CAD build for the part. Positions are in the model's coordinates, mm. A direction names the side the tool comes from. Coordinates: 2 decimals unless noted, no trailing zeros. Order: outer loops, then holes, each group sorted by start corner. A loop starts at its lowest first (then second) coordinate and runs counter-clockwise, first axis right, second up. Notation, with made-up numbers: M -31.75,38 L -18.75,38 A21 ccw -18.75,54 Z; hole C 62.5,22 d5. An arc over 180 degrees is marked long. One line per item, written item: value.
from build123d import *

# Parameters (mm, degrees)
F0_W     = 1500
F0_H     = 700
F1_DEPTH = 40
F2_W     = 300
F2_H     = 500
F3_DEPTH = 700
F4_W     = 420
F4_H     = 620
F5_DEPTH = 1328


with BuildPart() as f1:
    # F0 (on Top) → F1 (new body)
    with BuildSketch(Plane.XY):
        with Locations((750, -350)):
            Rectangle(F0_W, F0_H)
    extrude(amount=-F1_DEPTH)

    # F2 (on face) → F3 (join)
    with BuildSketch(Plane(origin=(0, 0, -40), x_dir=(1, 0, 0), z_dir=(0, 0, -1))):
        with Locations((250, 350)):
            Rectangle(F2_W, F2_H)
        with Locations((1250, 350)):
            Rectangle(F2_W, F2_H)
    extrude(amount=F3_DEPTH)

    # F4 (on face) → F5 (cut)
    with BuildSketch(Plane(origin=(100, 0, 0), x_dir=(0, -1, 0), z_dir=(-1, 0, 0))):
        with Locations((350, -390)):
            Rectangle(F4_W, F4_H)
    extrude(amount=-F5_DEPTH, mode=Mode.SUBTRACT)


solid = f1.part
Q1. Pin check, flat tips, straight feed: pin 1 Ø1 at (x, z) = (1127, -99.5) entering from +Y; pin 2 Ø3 at (x, y) = (482, -475) entering from -Z; pin 3 Ø1 at (x, y) = (496, -418.5) entering from +Z. Stop position of each tip, or through.
Recorded:
pin 1: stops at y = -100
pin 2: stops at z = -40
pin 3: stops at z = 0
Q2. Slice it at D-D (x = 338). List the corners of the cut face in (y, z), plus the area to 3 significant figures.
Recorded:
outline: M -700,-40 L -600,-40 L -600,-740 L -100,-740 L -100,-40 L 0,-40 L 0,0 L -700,0 Z; hole M -560,-700 L -140,-700 L -140,-80 L -560,-80 Z
area: 118,000 mm^2
Q3. Which spindle directions (+Z, -Z, +X, -X, +Y, -Y) get a long thin tool onto all of the face, cutting with end or side? Do faces 4 (the face through (740, -700, -20)), 5 (the face through (248, -100, -385)), 6 (the face through (1248, -600, -385)), 7 (the face through (248, -347, -700)), 8 (the face through (1100, -127, -362)). Say none if no direction does.
Recorded:
face 4: +Z, -Z, +X, -X, -Y
face 5: -Z, +X, -X, +Y
face 6: -Z, +X, -X, -Y
face 7: +X, -X
face 8: -Z, +Y, -Y
Q4. Drill centre lines: line 1 along Y through (x, z) = (195.5, -242); line 2 along Z through (x, y) = (267, -293.5); line 3 along Z through (x, y) = (902.5, -162). Where is each one in solid material? Low to high.
Recorded:
line 1: y = -600 to -560, -140 to -100
line 2: z = -740 to -700, -80 to 0
line 3: z = -40 to 0
Q5. Slice it at C-C (y = -542). List the corners of the cut face in (x, z).
Recorded:
outline: M 0,-40 L 100,-40 L 100,-80 L 400,-80 L 400,-40 L 1100,-40 L 1100,-80 L 1400,-80 L 1400,-40 L 1500,-40 L 1500,0 L 0,0 Z; M 100,-740 L 400,-740 L 400,-700 L 100,-700 Z; M 1100,-740 L 1400,-740 L 1400,-700 L 1100,-700 Z
Q6. Slice it at B-B (z = -556). List the corners of the cut face in (x, y).
Recorded:
outline: M 100,-600 L 400,-600 L 400,-560 L 100,-560 Z; M 100,-140 L 400,-140 L 400,-100 L 100,-100 Z; M 1100,-600 L 1400,-600 L 1400,-560 L 1100,-560 Z; M 1100,-140 L 1400,-140 L 1400,-100 L 1100,-100 Z
Q7. Slice it at A-A (z = -62.5). List the corners of the cut face in (x, y).
Recorded:
outline: M 100,-600 L 400,-600 L 400,-100 L 100,-100 Z; M 1100,-600 L 1400,-600 L 1400,-100 L 1100,-100 Z
Q8. Mould opens along X. For faces 1 (the face through (248, -354, -740)), 2 (the face through (0, -355, -20)), 3 (the face through (400, -127, -362)) say: released by +X, released by -X, zero draft, split by the parting line, or undercut.
Recorded:
face 1: zero draft
face 2: released by -X
face 3: undercut
